Can you work these out from the drawing? Everything is in mm from the part's minimum corner. A direction names the side the tool comes from. Round coordinates to 2 decimals unless told otherwise and drop trailing zeros. Write each loop counter-clockwise with the first axis right and the second up, starting at its lowest first coordinate (ties: lowest second). Pieces come first, ordered by that corner, then holes. Notation, with made-up numbers: M -8,-35 L 22,-35 A15 cw 22,-11 Z; hole C 61.25,45 d1. An arc over 180 degrees is marked long. Use a Markdown table: item, result. Add a question column.
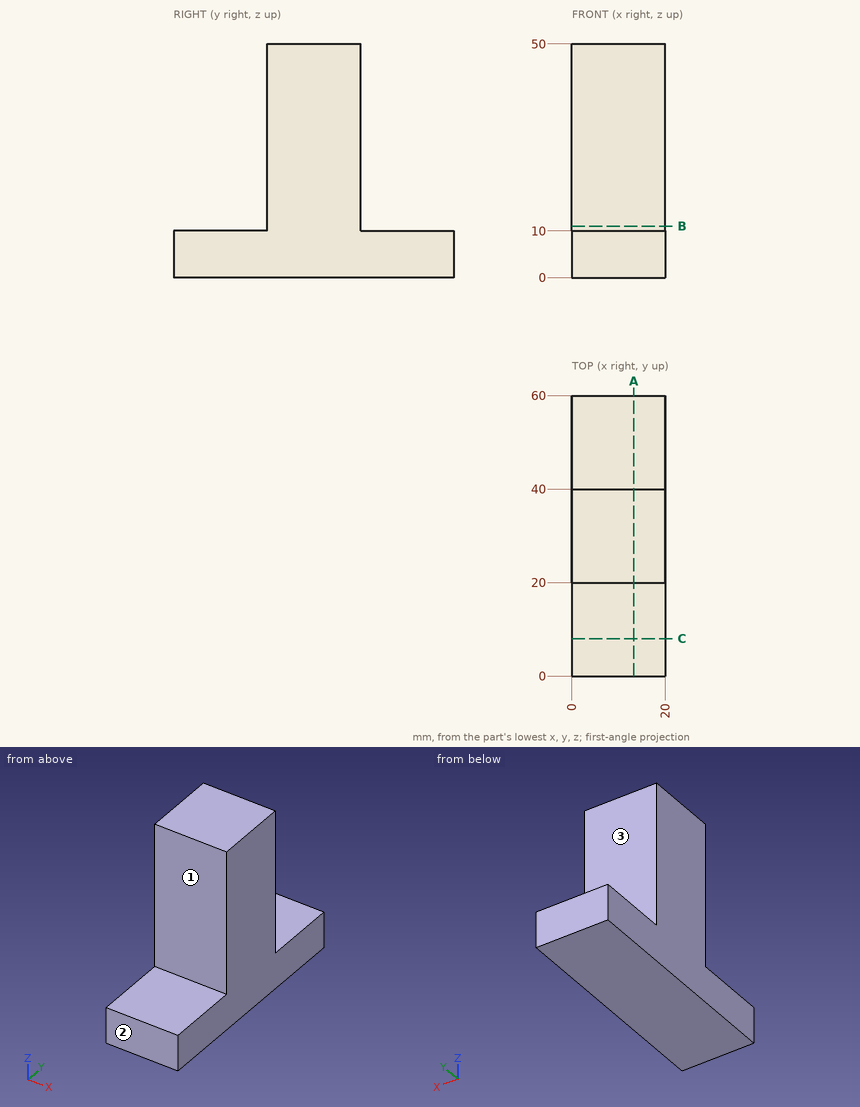
Item 1: Imagine slicing it at A-A on x = 13.25. List the corners of the cut face in (y, z) for me, plus the area to 3 significant figures.
Item 2: Imagine slicing it at B-B on z = 11. List the corners of the cut face in (x, y) for me.
Item 3: On a 3-axis mill with a long thin cutter (end or side, diameter ignored), from which of +Z, -Z, +X, -X, +Y, -Y can I reach the whole of each face in a straight line? I mean the marked faces 1, 2 and 3. Say none if no direction works.
Item 4: For pin 1 Ø1 at (x, z) = (11.5, 12.5) entering from +Y; pin 2 Ø8 at (x, y) = (5, 35) entering from -Z; pin 3 Ø10 at (x, z) = (2.5, 39) entering from -Y, each with a flat end and sliding along its axis, tell me the tip position at first contact or that it passes through.
Item 5: I need wall thicknesses on probe 1 along Z at (x, y) = (2, 40.5); probe 2 along Y at (x, z) = (10.75, 20.5). Which ranges of each line are inside material? Lowest first, please. Write a range as from..to.
Item 6: Imagine slicing it at C-C on y = 8. List the corners of the cut face in (x, z) for me.
The answers:
| question | item | result |
|---|---|---|
| 1 | outline | M 0,0 L 60,0 L 60,10 L 40,10 L 40,50 L 20,50 L 20,10 L 0,10 Z |
| 1 | area | 1,400 mm² |
| 2 | outline | M 0,20 L 20,20 L 20,40 L 0,40 Z |
| 3 | face 1 | +Z, +X, -X, -Y |
| 3 | face 2 | +Z, -Z, +X, -X, -Y |
| 3 | face 3 | +Z, +X, -X, +Y |
| 4 | pin 1 | y = 40 |
| 4 | pin 2 | z = 0 |
| 4 | pin 3 | y = 20 |
| 5 | probe 1 | 0..10 |
| 5 | probe 2 | 20..40 |
| 6 | outline | M 0,0 L 20,0 L 20,10 L 0,10 Z |
